Geometry: final body of the model. Coordinates: model frame, mm. A direction names the side the tool comes from. Give positions to 0.01 mm unless a question says otherwise; leave off trailing zeros. Order: outer loops, then holes, each group sorted by start corner. A loop starts at its lowest first (then second) coordinate and runs counter-clockwise, first axis right, second up. Notation, with made-up numbers: (8.5, -18) -> (61.5, -18) arc R28 ccw to (61.5, 13) -> close; hole circle Ø9 at (-22.75, 74.25). An arc over 180 degrees is marked (long way). Answer in a Markdown table with one row per item. Add a question column.
Q1. Cut plane D-D on y = 7. Return the cut outline in (x, z).
Q2. Cut plane A-A on z = -34. Return the cut outline in (x, y).
Q3. Pull-direction query (Y, two-part tool) for faces 1 (the face through (0, 0, -10)), 2 (the face through (11.503, -19.961, -20.28)), 3 (the face through (5, 0, 0)), 4 (the face through (0, -25, -20)); classes: +Y half, -Y half, draft (parallel to the pull), parting line (faces both ways), or undercut.
Q4. Contact query for flat-ended pins moving along their axis: P1, Ø3, axis at y = -10.5, z = -8, coming from the +X side; P2, Ø1, axis at y = -11.5, z = -14.5, coming from the -X side; P3, Ø2, axis at x = 5, z = -10, coming from the -Y side. Output: stop coordinate, or through.
Q5. Line query: line 1 along Y through (x, z) = (0, -38); line 2 along X through (y, z) = (-5.5, -24.5); line 3 along X through (y, z) = (10.5, -30). Output: solid intervals per line, ascending. Write a range as from..to.
Q6. Cut plane C-C on z = -3.5. Return the cut outline in (x, y).
Q7. Set-up query: faces 5 (the face through (21.711, 12.394, -19.72)), 6 (the face through (0, 3.25, -5)), 7 (the face through (0.267, 2.033, -35.07)). Return all of +Z, -Z, +X, -X, +Y, -Y with unobstructed straight access to the full face (end or side cutting, diameter ignored); none if empty.
Q8. Cut plane B-B on x = 0. Return the cut outline in (y, z), and give its area (3 significant figures).
from build123d import *

# Parameters (mm, degrees)
SKETCH1_R           = 25
BOSS_EXTRUDE1_DEPTH = 40
CUT_EXTRUDE1_DEPTH  = 54.38539126
CIRPATTERN1_START   = -40
CIRPATTERN1_DEPTH   = 40
CUT_EXTRUDE2_DEPTH  = 10
SKETCH4_R           = 2.05
CUT_EXTRUDE3_DEPTH  = 10


# Read off the part's stored shape, not the designer's step: CirPattern1
with BuildPart() as part:
    # Sketch1 → Boss-Extrude1 (new body)
    with BuildSketch(Plane.XY):
        Circle(SKETCH1_R)
    extrude(amount=-BOSS_EXTRUDE1_DEPTH)

    # Sketch2 → Cut-Extrude1 (cut, through all)
    with BuildSketch(Plane.XY):
        with BuildLine():
            Line((148.327454228, 6.938651312), (24.92, 1.998399359))
            ThreePointArc((24.92, 1.998399359), (23, 0), (24.92, -1.998399359))
            Line((24.92, -1.998399359), (148.327454228, -6.938651312))
            Line((148.327454228, -6.938651312), (395.340051868, -6.938651312))
            Line((395.340051868, -6.938651312), (395.340051868, 6.938651312))
            Line((395.340051868, 6.938651312), (148.327454228, 6.938651312))
        make_face()
    extrude(amount=-CUT_EXTRUDE1_DEPTH, mode=Mode.SUBTRACT)

    # CirPattern1 outline → CirPattern1 (cut)
    with BuildSketch(Plane.XY.offset(CIRPATTERN1_START)):
        with BuildLine():
            ThreePointArc((14.134833251, -20.620535613), (11.466483325, -19.981917804), (10.671520375, -22.607933406))
            ThreePointArc((10.671520375, -22.607933406), (12.442918972, -21.683490666), (14.134833251, -20.620535613))
        make_face()
        with BuildLine():
            ThreePointArc((-10.795666007, -22.548915616), (-11.609703747, -19.987178691), (-14.238240755, -20.549270065))
            ThreePointArc((-14.238240755, -20.549270065), (-12.556821553, -21.617729586), (-10.795666007, -22.548915616))
        make_face()
        with BuildLine():
            ThreePointArc((-24.920945806, -1.986569943), (-23.152332628, 0), (-24.920945806, 1.986569943))
            ThreePointArc((-24.920945806, 1.986569943), (-25, 0), (-24.920945806, -1.986569943))
        make_face()
        with BuildLine():
            ThreePointArc((-14.238240755, 20.549270065), (-11.609703747, 19.987178691), (-10.795666007, 22.548915616))
            ThreePointArc((-10.795666007, 22.548915616), (-12.556821553, 21.617729586), (-14.238240755, 20.549270065))
        make_face()
        with BuildLine():
            ThreePointArc((10.671520375, 22.607933406), (11.466483325, 19.981917804), (14.134833251, 20.620535613))
            ThreePointArc((14.134833251, 20.620535613), (12.442918972, 21.683490666), (10.671520375, 22.607933406))
        make_face()
    extrude(amount=CIRPATTERN1_DEPTH, mode=Mode.SUBTRACT)

    # Sketch3 → Cut-Extrude2 (cut)
    with BuildSketch(Plane.XY):
        Polygon((3.75277675, 0), (1.876388375, 3.25), (-1.876388375, 3.25), (-3.75277675, 0), (-1.876388375, -3.25), (1.876388375, -3.25), align=None)
    extrude(amount=-CUT_EXTRUDE2_DEPTH, mode=Mode.SUBTRACT)

    # Sketch4 → Cut-Extrude3 (cut)
    with BuildSketch(Plane(origin=(0, 0, -40), x_dir=(-1, 0, 0), z_dir=(0, 0, -1))):
        Circle(SKETCH4_R)
    extrude(amount=-CUT_EXTRUDE3_DEPTH, mode=Mode.SUBTRACT)


solid = part.part
Completed:
| question | item | result |
|---|---|---|
| 1 | outline | (-24, -40) -> (24, -40) -> (24, 0) -> (-24, 0) -> close |
| 2 | outline | (-24.92, -1.99) arc R25 ccw to (-14.24, -20.55) arc R2 cw to (-10.8, -22.55) arc R25 ccw to (10.67, -22.61) arc R2 cw to (14.13, -20.62) arc R25 ccw to (24.92, -2) arc R2 cw to (24.92, 2) arc R25 ccw to (14.13, 20.62) arc R2 cw to (10.67, 22.61) arc R25 ccw to (-10.8, 22.55) arc R2 cw to (-14.24, 20.55) arc R25 ccw to (-24.92, 1.99) arc R2 cw to start; hole circle Ø4.1 at (0, 0) |
| 3 | face 1 | undercut |
| 3 | face 2 | undercut |
| 3 | face 3 | draft |
| 3 | face 4 | -Y half |
| 4 | P1 | stops at x = 23.32 |
| 4 | P2 | stops at x = -22.45 |
| 4 | P3 | stops at y = -24.68 |
| 5 | line 1 | y = -25..-2.05, 2.05..25 |
| 5 | line 2 | x = -24.39..24.39 |
| 5 | line 3 | x = -22.69..22.69 |
| 6 | outline | (-24.92, -1.99) arc R25 ccw to (-14.24, -20.55) arc R2 cw to (-10.8, -22.55) arc R25 ccw to (10.67, -22.61) arc R2 cw to (14.13, -20.62) arc R25 ccw to (24.92, -2) arc R2 cw to (24.92, 2) arc R25 ccw to (14.13, 20.62) arc R2 cw to (10.67, 22.61) arc R25 ccw to (-10.8, 22.55) arc R2 cw to (-14.24, 20.55) arc R25 ccw to (-24.92, 1.99) arc R2 cw to start; hole (-3.75, 0) -> (-1.88, -3.25) -> (1.88, -3.25) -> (3.75, 0) -> (1.88, 3.25) -> (-1.88, 3.25) -> close |
| 7 | face 5 | +Z, -Z, +X, +Y |
| 7 | face 6 | +Z |
| 7 | face 7 | -Z |
| 8 | outline | (-25, -40) -> (-2.05, -40) -> (-2.05, -30) -> (2.05, -30) -> (2.05, -40) -> (25, -40) -> (25, 0) -> (3.25, 0) -> (3.25, -10) -> (-3.25, -10) -> (-3.25, 0) -> (-25, 0) -> close |
| 8 | area | 1,890 mm² |
